Model file for the job. Use its own axes, mm. A direction names the side the tool comes from. Coordinates: 2 decimals unless noted, no trailing zeros. Write each loop counter-clockwise with the first axis right and the second up, starting at its lowest first coordinate (ties: lowest second). Pieces come first, ordered by that corner, then holes. Notation, with made-up numbers: M 70,74.5 L 120,74.5 A23 cw 120,87.5 Z; hole C 58.5,29.25 d11. An arc over 180 degrees is marked long. Use CSV: the item, a comma, the result in double quotes. Start each with the question number.
Autodesk Inventor part; units mm, degrees
ref_plane "YZ Plane" through (0, 0, 0) normal (1, 0, 0) x (0, 1, 0)
ref_plane "XZ Plane" through (0, 0, 0) normal (0, 1, 0) x (-1, 0, 0)
ref_plane "XY Plane" through (0, 0, 0) normal (0, 0, 1) x (1, 0, 0)
sketch "Sketch1" plane through (0, 0, 0) normal (0, 0, 1) x (1, 0, 0)
  arc A0 (21.2132, 1.5875) -> (21.2132, -1.5875) centre (0, 0) ccw
  arc A1 (0, 33.9725) -> (-33.9725, 0) centre (0, 0) ccw
  line L0 (0, -33.9725) -> (-33.9725, -33.9725)
  line L1 (-33.9725, 0) -> (-33.9725, -33.9725)
  line L2 (0, 33.9725) -> (33.9725, 33.9725)
  line L3 (0, -33.9725) -> (33.9725, -33.9725)
  line L4 (33.9725, 0) -> (33.9725, -33.9725)
  line L5 (33.9725, 0) -> (33.9725, 33.9725)
  line L6 (0, 0) -> (24.13, 0) construction
  line L7 (21.2132, 1.5875) -> (22.8007, 1.5875)
  line L8 (22.8007, 1.5875) -> (22.8007, -1.5875)
  line L9 (22.8007, -1.5875) -> (21.2132, -1.5875)
  dimension "d0" = 42.545
  dimension "d1" = 67.945
  dimension "d22" = 1.5875
  dimension "d23" = 1.5875
  dimension "d24" = 1.5875
extrude "Extrusion1" add sketch "Sketch1" along normal mid plane 38.1
sketch "Sketch2" plane through (-33.9725, -33.9725, 19.05) normal (-1, 0, 0) x (0, 0, 1)
  line L0 (0, 0) -> (-38.1, 0) construction
  line L1 (-19.05, 0) -> (-19.05, 33.9725) construction
  point P0 (-19.05, 10.16)
  dimension "d4" = 10.16
hole "Hole1" at (-33.9725, -23.8125, 0) direction (1, 0, 0) diameter 4.9784 depth 31.75 tip angle 118
sketch "Sketch3" plane through (33.9725, -33.9725, 19.05) normal (1, 0, 0) x (0, 0, -1)
  line L0 (0, 67.945) -> (38.1, 67.945) construction
  line L1 (19.05, 67.945) -> (19.05, 0) construction
  line L2 (0, 0) -> (38.1, 0) construction
  line L3 (6.35, 67.945) -> (6.35, 0) construction
  line L4 (31.75, 67.945) -> (31.75, 0) construction
  line L5 (0, 0) -> (0, 67.945) construction
  line L6 (38.1, 67.945) -> (38.1, 0) construction
  point P0 (19.05, 33.9725)
  point P1 (19.05, 61.595)
  point P2 (19.05, 6.35)
  point P3 (6.35, 61.595)
  point P4 (31.75, 61.595)
  point P5 (31.75, 6.35)
  point P6 (6.35, 6.35)
  dimension "d13" = 6.35
  dimension "d14" = 6.35
  dimension "d25" = 6.35
  dimension "d26" = 6.35
  dimension "d27" = 6.35
  dimension "d28" = 6.35
  dimension "d29" = 6.35
split "Split1" plane through (0, 0, 0) removes the side toward (-1, 0, 0)
hole "Hole2" at (33.9725, 27.6225, 0) at (33.9725, -27.6225, 0) at (33.9725, 27.6225, 12.7) at (33.9725, 27.6225, -12.7) at (33.9725, -27.6225, -12.7) at (33.9725, -27.6225, 12.7) direction (-1, 0, 0) diameter 6.6294 end through all
equation "\"d0\" = pipeDiameter"
equation "\"d1\" = pipeDiameter + 2 * outerRadius"
equation "\"d2\" = width"
equation "\"pipeDiameter\" = 42.545"
equation "\"outerRadius\" = 12.7"
equation "\"width\" = 38.1"
properties part number "gripperBracketB" material "Aluminum 6061"
1) Drop flat-ended pins along their axis: P1, Ø2.5, axis at y = 0, z = -7, coming from the -X side; P2, Ø12, axis at y = 9, z = -10.5, coming from the -X side; P3, Ø12, axis at y = -6.5, z = -8, coming from the -X side. Give the stop position or say it passes through.
2) Band-saw the part on D-D on z = 14. List the corners of the cut face in (x, y), then the cut area to 3 significant figures.
3) Band-saw the part on B-B on z = 0. List the corners of the cut face in (x, y).
4) Band-saw the part on A-A on x = 20. List the corners of the cut face in (y, z), then the cut area to 3 significant figures.
5) Two-plate mould, pull along Z, no slides. Class faces 1 (the face through (16.748, -25.606, -10.07)), 2 (the face through (22.801, 0, 0)), 3 (the face through (24, 0, 19.05)), 4 (the face through (16.75, 29.64, -10.07)): pulls with the +Z half, pulls with the -Z half, needs draft (parallel to the pull), parting line crosses it, or undercut.
6) Band-saw the part on C-C on x = 26. List the corners of the cut face in (y, z).
7) Tool access for faces 5 (the face through (22, 1.588, 0)), 6 (the face through (17, 33.972, 0)): list every direction of +Z, -Z, +X, -X, +Y, -Y with a clear straight run to the whole face (end or side of a thin tool).
8) Wall check: L1, parallel to Y at x = 14, z = 0; L2, parallel to Y at x = 22, z = 14; L3, parallel to Y at x = 24, z = 13.5. Give the ranges that are in metal, low to high. Write a range as [from, to].
Findings below:
1,P1,"stops at x = 22.8"
1,P2,"stops at x = 15.08"
1,P3,"stops at x = 17.21"
2,outline,"M 0,-33.97 L 33.97,-33.97 L 33.97,-30.67 L 0,-30.67 Z; M 0,-24.57 L 33.97,-24.57 L 33.97,24.57 L 0,24.57 L 0,21.27 A21.27 cw 21.21,1.59 L 22.8,1.59 L 22.8,-1.59 L 21.21,-1.59 A21.27 cw 0,-21.27 Z; M 0,30.67 L 33.97,30.67 L 33.97,33.97 L 0,33.97 Z"
2,area,"1,180 mm2"
3,outline,"M 0,-33.97 L 33.97,-33.97 L 33.97,-30.94 L 0,-30.94 Z; M 0,-24.31 L 33.97,-24.31 L 33.97,24.31 L 0,24.31 L 0,21.27 A21.27 cw 21.21,1.59 L 22.8,1.59 L 22.8,-1.59 L 21.21,-1.59 A21.27 cw 0,-21.27 Z; M 0,30.94 L 33.97,30.94 L 33.97,33.97 L 0,33.97 Z"
4,outline,"M -33.97,-19.05 L -7.25,-19.05 L -7.25,19.05 L -33.97,19.05 Z; M 7.25,-19.05 L 33.97,-19.05 L 33.97,19.05 L 7.25,19.05 Z; hole C -27.62,-12.7 d6.63; hole C -27.62,0 d6.63; hole C -27.62,12.7 d6.63; hole C 27.62,-12.7 d6.63; hole C 27.62,0 d6.63; hole C 27.62,12.7 d6.63"
4,area,"1,830 mm2"
5,face 1,"undercut"
5,face 2,"needs draft"
5,face 3,"pulls with the +Z half"
5,face 4,"undercut"
6,outline,"M -33.97,-19.05 L 33.97,-19.05 L 33.97,19.05 L -33.97,19.05 Z; hole C -27.62,-12.7 d6.63; hole C -27.62,0 d6.63; hole C -27.62,12.7 d6.63; hole C 27.62,-12.7 d6.63; hole C 27.62,0 d6.63; hole C 27.62,12.7 d6.63"
7,face 5,"+Z, -Z, -X"
7,face 6,"+Z, -Z, +X, -X, +Y"
8,L1,"y = [-33.97, -30.94], [-24.31, -16.02], [16.02, 24.31], [30.94, 33.97]"
8,L2,"y = [-33.97, -30.67], [-24.57, -1.59], [1.59, 24.57], [30.67, 33.97]"
8,L3,"y = [-33.97, -30.84], [-24.41, 24.41], [30.84, 33.97]"
